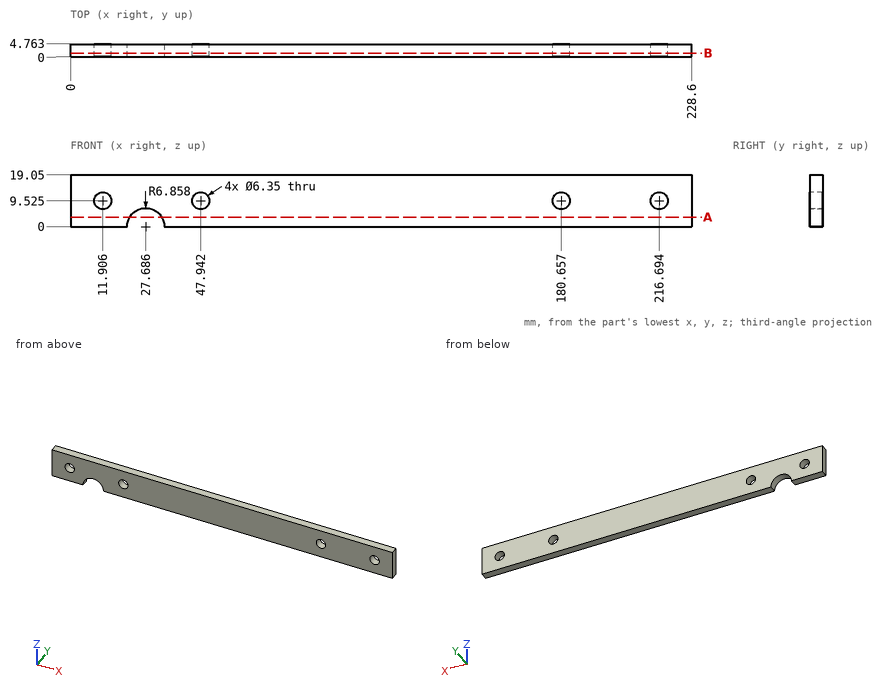
Input: dimensioned drawing with shaded views. Units: mm. Origin: part minimum x, y, z. Coordinates: 2 decimals unless noted, no trailing zeros. Order: outer loops, then holes, each group sorted by start corner. A loop starts at its lowest first (then second) coordinate and runs counter-clockwise, first axis right, second up. Notation, with made-up numbers: (78.5, 39.5) - (123.5, 39.5) arc R18 cw to (123.5, 64.5) - close; hole circle Ø11 at (24.25, 49.5). An arc over 180 degrees is marked (long way). One line per item, written item: value.
1) Ray query, line 1 (X direction, y = 1.8, z = 9) (1 decimal); line 2 (X direction, y = 1.4, z = 11.5) (1 decimal); line 3 (X direction, y = 0.75, z = 1). Return the intervals inside material, ascending. Write a range as [from, to].
Computed values:
line 1: x = [0, 8.8], [15, 44.8], [51.1, 177.5], [183.8, 213.6], [219.8, 228.6]
line 2: x = [0, 9.4], [14.4, 45.5], [50.4, 178.2], [183.1, 214.2], [219.2, 228.6]
line 3: x = [0, 20.9], [34.47, 228.6]
2) Cut plane A-A on z = 3.5. Output: boundary loops of the cut face in (x, y), plus the area to 3 significant figures.
Computed values:
outline: (0, 0) - (21.79, 0) - (21.79, 4.76) - (0, 4.76) - close; (33.58, 0) - (228.6, 0) - (228.6, 4.76) - (33.58, 4.76) - close
area: 1,030 mm^2
3) Cut plane B-B on y = 1.4. State how many separate pieces and enclosed holes the cut face has, plus the area to 3 significant figures.
Computed values:
separate pieces: 1
enclosed holes: 4
area: 4,150 mm^2
